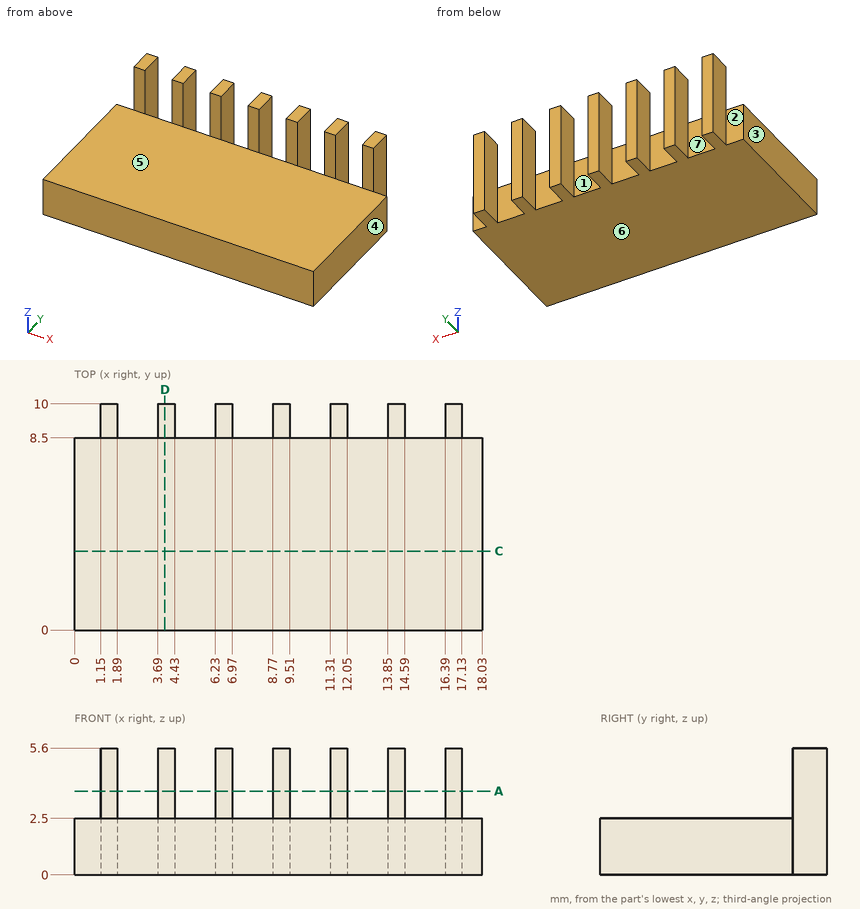
The drawing under review shows one solid part. Ordinate dimensions are in mm from its lowest x, y, z. A direction names the side the tool comes from. Coordinates: 2 decimals unless noted, no trailing zeros. Write each loop counter-clockwise with the first axis right and the second up, starting at its lowest first coordinate (ties: lowest second). Pieces come first, ordered by that corner, then holes. Notation, with made-up numbers: M 34.25,-39.5 L 74.25,-39.5 A19 cw 74.25,-26.5 Z; hole C 23.25,11.5 d10. An arc over 180 degrees is marked long. Put each result on its own line as item: value.
1) Draft analysis for pull direction X (two halves, no side actions). For the marked faces 1, 2, 3 and 4, state which applies: released by +X, released by -X, zero draft, split by the parting line, or undercut.
Computed:
face 1: undercut
face 2: zero draft
face 3: released by -X
face 4: released by +X
2) Clearance check with flat-ended pins moving along their axes: pin 1 Ø0.6 at (x, z) = (0.5, 1) entering from +Y; pin 2 Ø1.2 at (y, z) = (9, 1.5) entering from +X; pin 3 Ø0.6 at (x, z) = (12, 3.5) entering from -Y; pin 4 Ø3 at (x, y) = (14.5, 1) entering from +Z. State where each tip first meets the part, or that it passes through.
Computed:
pin 1: stops at y = 8.5
pin 2: stops at x = 18.03
pin 3: stops at y = 8.5
pin 4: stops at z = 2.5
3) Wall thickness on probe 1 along Z at (x, y) = (16, 4.5); probe 2 along Y at (x, z) = (7, 0.65); probe 3 along Y at (x, z) = (6.5, 5): over which ranges is each line inside the solid? List them lowest first. Write a range as [from, to].
Computed:
probe 1: z = [0, 2.5]
probe 2: y = [0, 8.5]
probe 3: y = [8.5, 10]
4) For the marked faces 5, 6 and 7, list the 3-axis set-ups (+Z, -Z, +X, -X, +Y, -Y) from which the entire face can be reached by the end or side of a thin tool; tool diameter is ignored.
Computed:
face 5: +Z, +X, -X, -Y
face 6: -Z, +X, -X, +Y, -Y
face 7: +Z, -Z, +Y
5) Add section D-D on x = 4. Give the boundary of the cut face in (y, z).
Computed:
outline: M 0,0 L 10,0 L 10,5.6 L 8.5,5.6 L 8.5,2.5 L 0,2.5 Z
6) Add section C-C on y = 3.5. Give the boundary of the cut face in (x, z), then the cut area to 3 significant figures.
Computed:
outline: M 0,0 L 18.03,0 L 18.03,2.5 L 0,2.5 Z
area: 45.1 mm2
7) Add section A-A on z = 3.7. Give the boundary of the cut face in (x, y), then the cut area to 3 significant figures.
Computed:
outline: M 1.15,8.5 L 1.89,8.5 L 1.89,10 L 1.15,10 Z; M 3.69,8.5 L 4.43,8.5 L 4.43,10 L 3.69,10 Z; M 6.23,8.5 L 6.97,8.5 L 6.97,10 L 6.23,10 Z; M 8.77,8.5 L 9.51,8.5 L 9.51,10 L 8.77,10 Z; M 11.31,8.5 L 12.05,8.5 L 12.05,10 L 11.31,10 Z; M 13.85,8.5 L 14.59,8.5 L 14.59,10 L 13.85,10 Z; M 16.39,8.5 L 17.13,8.5 L 17.13,10 L 16.39,10 Z
area: 7.77 mm2
